Design review of the part built by this model. Coordinates are the model's own, in mm. Face numbers are marked on the shaded views. A direction names the side the tool comes from. Round coordinates to 2 decimals unless told otherwise and drop trailing zeros. Order: outer loops, then holes, each group sorted by start corner. A loop starts at its lowest first (then second) coordinate and runs counter-clockwise, first axis right, second up. Notation, with made-up numbers: M 25.25,46.5 L 40.25,46.5 A8 cw 40.25,55.5 Z; hole C 50,86 d2. An arc over 180 degrees is marked long. Write each question's results on one line, items separated by ' | '. Start each with the question number.
Item 1: The part is to be moulded in two halves that separate along Y. For the marked faces 1, 2 and 3, say which applies: +Y half, -Y half, draft (parallel to the pull), parting line (faces both ways), or undercut.
Item 2: Wall thickness on line 1 (Y direction, x = 15, z = 3.25); line 2 (Z direction, x = 14.5, y = 3); line 3 (Z direction, x = 28.5, y = -6): over which ranges is each line inside the solid? List them lowest first. Write a range as [from, to].
Item 3: Clearance check with flat-ended pins moving along their axes: pin 1 (6 mm diameter, centred on x = -23.5, z = 6.5, fed in from +Y); pin 2 (1 mm diameter, centred on x = 14, y = 1, fed in from +Z); pin 3 (1.2 mm diameter, centred on y = -9.5, z = 3, fed in from -X); pin 4 (2 mm diameter, centred on y = -9, z = 7.5, fed in from -X). State where each tip first meets the part, or that it passes through.
Item 4: Take a section at D-D, the plane z = 3. Write out the cut boundary in (x, y) (3 decimals).
Item 5: Machinability: for the marked faces 4, 5 and 6, which of the approach directions +Z, -Z, +X, -X, +Y, -Y give a long, thin tool a straight path to every point of the face, cutting with its end or side? Answer none if there is none.
Item 6: Take a section at C-C, the plane x = -27. Write out the cut boundary in (y, z).
Item 7: Take a section at A-A, the plane y = 1.25. Write out the cut boundary in (x, z), plus the area to 3 significant figures.
Item 8: Take a section at B-B, the plane z = 6. Write out the cut boundary in (x, y), plus the area to 3 significant figures.
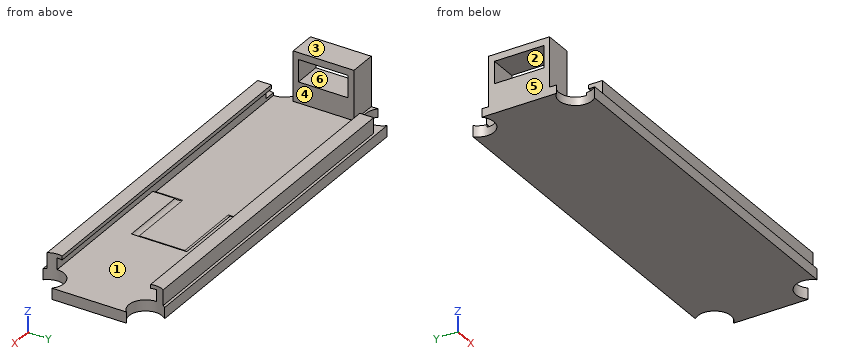
```python
from build123d import *

# Parameters (mm, degrees)
SKIZZE1_W                       = 22
SKIZZE1_H                       = 72.8
AUFSATZ_LINEAR_AUSTRAGEN1_DEPTH = 2
SKIZZE2_R                       = 3
SCHNITT_LINEAR_AUSTRAGEN1_DEPTH = 2
SKIZZE3_W                       = 65.5
SKIZZE3_H                       = 21
AUFSATZ_LINEAR_AUSTRAGEN2_DEPTH = 2.8
SCHNITT_LINEAR_AUSTRAGEN2_DEPTH = 67.590464783
SKIZZE5_R                       = 3
SCHNITT_LINEAR_AUSTRAGEN4_DEPTH = 39.128729326
SKIZZE6_W                       = 18
SKIZZE6_H                       = 1
SCHNITT_LINEAR_AUSTRAGEN5_DEPTH = 40
SKIZZE8_W                       = 15
SKIZZE8_H                       = 10
SCHNITT_LINEAR_AUSTRAGEN6_DEPTH = 0.5
VERRUNDUNG3_R                   = 1
SKIZZE9_W                       = 5
SKIZZE9_H                       = 11
AUFSATZ_LINEAR_AUSTRAGEN3_DEPTH = 9
SKIZZE10_W                      = 9
SKIZZE10_H                      = 4
SCHNITT_LINEAR_AUSTRAGEN7_DEPTH = 75.371298227


with BuildPart() as part:
    # Skizze1 → Aufsatz-Linear austragen1 (new body)
    with BuildSketch(Plane(origin=(0, 0, 0), x_dir=(0, 1, 0), z_dir=(0, 0, 1))):
        Rectangle(SKIZZE1_W, SKIZZE1_H)
    extrude(amount=AUFSATZ_LINEAR_AUSTRAGEN1_DEPTH)

    # Skizze2 → Schnitt-Linear austragen1 (cut)
    with BuildSketch(Plane.XY.offset(2)):
        with Locations((-34.28, 8.88)):
            Circle(SKIZZE2_R)
        with Locations((-34.28, -8.88)):
            Circle(SKIZZE2_R)
        with Locations((34.28, -8.88)):
            Circle(SKIZZE2_R)
        with Locations((34.28, 8.88)):
            Circle(SKIZZE2_R)
    extrude(amount=-SCHNITT_LINEAR_AUSTRAGEN1_DEPTH, mode=Mode.SUBTRACT)

    # Skizze3 → Aufsatz-Linear austragen2 (add)
    with BuildSketch(Plane.XY.offset(2)):
        with Locations((3.65, 0)):
            Rectangle(SKIZZE3_W, SKIZZE3_H)
    extrude(amount=AUFSATZ_LINEAR_AUSTRAGEN2_DEPTH)

    # Skizze4 → Schnitt-Linear austragen2 (cut, through all)
    with BuildSketch(Plane(origin=(-29.1, 0, 0), x_dir=(0, -1, 0), z_dir=(-1, 0, 0))):
        Polygon((-8, 4.8), (8, 4.8), (8, 4.1), (9, 4.1), (9, 2), (-9, 2), (-9, 4.1), (-8, 4.1), align=None)
    extrude(amount=-SCHNITT_LINEAR_AUSTRAGEN2_DEPTH, mode=Mode.SUBTRACT)

    # Skizze5 → Schnitt-Linear austragen4 (cut, through all)
    with BuildSketch(Plane(origin=(0, 0, 2), x_dir=(1, 0, 0), z_dir=(0, 0, -1))):
        with Locations((34.28, -8.88)):
            Circle(SKIZZE5_R)
        with Locations((34.28, 8.88)):
            Circle(SKIZZE5_R)
    extrude(amount=-SCHNITT_LINEAR_AUSTRAGEN4_DEPTH, mode=Mode.SUBTRACT)

    # Skizze6 → Schnitt-Linear austragen5 (cut)
    with BuildSketch(Plane(origin=(-36.4, 0, 0), x_dir=(0, -1, 0), z_dir=(-1, 0, 0))):
        with Locations((0, 2)):
            Rectangle(SKIZZE6_W, SKIZZE6_H)
    extrude(amount=-SCHNITT_LINEAR_AUSTRAGEN5_DEPTH, mode=Mode.SUBTRACT)

    # Skizze8 → Schnitt-Linear austragen6 (cut)
    with BuildSketch(Plane.XY.offset(2)):
        with Locations((8.655984658, -0.007335612)):
            Rectangle(SKIZZE8_W, SKIZZE8_H)
    extrude(amount=-SCHNITT_LINEAR_AUSTRAGEN6_DEPTH, mode=Mode.SUBTRACT)

    # Verrundung3
    # the kernel refuses this fillet: 1 mm, written as the material it adds along each edge
    with BuildSketch(Plane(origin=(3.6, -9, 1.5), x_dir=(0, 0, 1), z_dir=(0, 1, 0))) as verrundung3_piece_1:
        with BuildLine():
            CenterArc((1, -0.866025404), VERRUNDUNG3_R, 120, 60)
            Line((0, -0.866025404), (-0.02, -0.866025404))
            Line((-0.02, -0.866025404), (-0.02, 0))
            Line((-0.02, 0), (0, 0.02))
            ThreePointArc((0, 0.02), (0.25, 0.02), (0.49, 0.017320508))
            Line((0.49, 0.017320508), (0.5, 0))
        make_face()
    extrude(amount=3.992664388)
    with BuildSketch(Plane(origin=(3.6, -5.007335612, 1.5), x_dir=(0, 0, 1), z_dir=(1, 0, 0)), Plane(origin=(16.155984658, 4.992664388, 1.5), x_dir=(0, 0, 1), z_dir=(-1, 0, 0))) as verrundung3_piece_2:
        with BuildLine():
            CenterArc((1, -0.866025404), VERRUNDUNG3_R, 120, 60)
            Line((0, -0.866025404), (-0.02, -0.866025404))
            Line((-0.02, -0.866025404), (-0.02, 0))
            Line((-0.02, 0), (0, 0.02))
            ThreePointArc((0, 0.02), (0.25, 0.02), (0.49, 0.017320508))
            Line((0.49, 0.017320508), (0.5, 0))
        make_face()
    extrude(amount=12.555984658)
    with BuildSketch(Plane(origin=(3.6, 4.992664388, 1.5), x_dir=(0, 0, 1), z_dir=(0, 1, 0))) as verrundung3_piece_3:
        with BuildLine():
            CenterArc((1, -0.866025404), VERRUNDUNG3_R, 120, 60)
            Line((0, -0.866025404), (-0.02, -0.866025404))
            Line((-0.02, -0.866025404), (-0.02, 0))
            Line((-0.02, 0), (0, 0.02))
            ThreePointArc((0, 0.02), (0.25, 0.02), (0.49, 0.017320508))
            Line((0.49, 0.017320508), (0.5, 0))
        make_face()
    extrude(amount=4.007335612)
    with BuildSketch(Plane(origin=(16.155984658, -5.007335612, 1.5), x_dir=(0, 0, 1), z_dir=(0, 1, 0))) as verrundung3_piece_4:
        with BuildLine():
            CenterArc((1, -0.866025404), VERRUNDUNG3_R, 120, 60)
            Line((0, -0.866025404), (-0.02, -0.866025404))
            Line((-0.02, -0.866025404), (-0.02, 0))
            Line((-0.02, 0), (0, 0.02))
            ThreePointArc((0, 0.02), (0.25, 0.02), (0.49, 0.017320508))
            Line((0.49, 0.017320508), (0.5, 0))
        make_face()
    extrude(amount=10)
    with BuildSketch(Plane(origin=(3.6, -9, 1.5), x_dir=(0, 0, 1), z_dir=(0, 1, 0))) as verrundung3_piece_5a_section:
        with BuildLine():
            CenterArc((1, -0.866025404), VERRUNDUNG3_R, 120, 60)
            Line((0, -0.866025404), (-0.02, -0.866025404))
            Line((-0.02, -0.866025404), (-0.02, 0))
            Line((-0.02, 0), (0, 0.02))
            ThreePointArc((0, 0.02), (0.25, 0.02), (0.49, 0.017320508))
            Line((0.49, 0.017320508), (0.5, 0))
        make_face()
    verrundung3_piece_5a = extrude(amount=6.157727897, mode=Mode.PRIVATE)
    verrundung3_piece_5a = split(verrundung3_piece_5a, bisect_by=Plane(origin=(3.383689554, -5.007335612, 1.629516711), z_dir=(0, 1, 0)), keep=Keep.TOP, mode=Mode.PRIVATE)
    with BuildSketch(Plane(origin=(1.434936491, -5.007335612, 1.5), x_dir=(0, 0, 1), z_dir=(1, 0, 0))) as verrundung3_piece_5b_section:
        with BuildLine():
            CenterArc((1, -0.866025404), VERRUNDUNG3_R, 120, 60)
            Line((0, -0.866025404), (-0.02, -0.866025404))
            Line((-0.02, -0.866025404), (-0.02, 0))
            Line((-0.02, 0), (0, 0.02))
            ThreePointArc((0, 0.02), (0.25, 0.02), (0.49, 0.017320508))
            Line((0.49, 0.017320508), (0.5, 0))
        make_face()
    verrundung3_piece_5b = extrude(amount=14.721048168, mode=Mode.PRIVATE)
    verrundung3_piece_5b = split(verrundung3_piece_5b, bisect_by=Plane(origin=(3.6, -4.791025166, 1.629516711), z_dir=(-1, 0, 0)), keep=Keep.TOP, mode=Mode.PRIVATE)
    verrundung3_piece_5 = verrundung3_piece_5a & verrundung3_piece_5b
    add(verrundung3_piece_5)
    with BuildSketch(Plane(origin=(3.6, -5.007335612, 1.5), x_dir=(0, 0, 1), z_dir=(1, 0, 0))) as verrundung3_piece_6a_section:
        with BuildLine():
            CenterArc((1, -0.866025404), VERRUNDUNG3_R, 120, 60)
            Line((0, -0.866025404), (-0.02, -0.866025404))
            Line((-0.02, -0.866025404), (-0.02, 0))
            Line((-0.02, 0), (0, 0.02))
            ThreePointArc((0, 0.02), (0.25, 0.02), (0.49, 0.017320508))
            Line((0.49, 0.017320508), (0.5, 0))
        make_face()
    verrundung3_piece_6a = extrude(amount=14.721048168, mode=Mode.PRIVATE)
    verrundung3_piece_6a = split(verrundung3_piece_6a, bisect_by=Plane(origin=(16.155984658, -4.791025166, 1.629516711), z_dir=(1, 0, 0)), keep=Keep.TOP, mode=Mode.PRIVATE)
    with BuildSketch(Plane(origin=(16.155984658, -7.172399122, 1.5), x_dir=(0, 0, 1), z_dir=(0, 1, 0))) as verrundung3_piece_6b_section:
        with BuildLine():
            CenterArc((1, -0.866025404), VERRUNDUNG3_R, 120, 60)
            Line((0, -0.866025404), (-0.02, -0.866025404))
            Line((-0.02, -0.866025404), (-0.02, 0))
            Line((-0.02, 0), (0, 0.02))
            ThreePointArc((0, 0.02), (0.25, 0.02), (0.49, 0.017320508))
            Line((0.49, 0.017320508), (0.5, 0))
        make_face()
    verrundung3_piece_6b = extrude(amount=12.165063509, mode=Mode.PRIVATE)
    verrundung3_piece_6b = split(verrundung3_piece_6b, bisect_by=Plane(origin=(15.939674213, -5.007335612, 1.629516711), z_dir=(0, -1, 0)), keep=Keep.TOP, mode=Mode.PRIVATE)
    verrundung3_piece_6 = verrundung3_piece_6a & verrundung3_piece_6b
    add(verrundung3_piece_6)
    with BuildSketch(Plane(origin=(16.155984658, 4.992664388, 1.5), x_dir=(0, 0, 1), z_dir=(-1, 0, 0))) as verrundung3_piece_7a_section:
        with BuildLine():
            CenterArc((1, -0.866025404), VERRUNDUNG3_R, 120, 60)
            Line((0, -0.866025404), (-0.02, -0.866025404))
            Line((-0.02, -0.866025404), (-0.02, 0))
            Line((-0.02, 0), (0, 0.02))
            ThreePointArc((0, 0.02), (0.25, 0.02), (0.49, 0.017320508))
            Line((0.49, 0.017320508), (0.5, 0))
        make_face()
    verrundung3_piece_7a = extrude(amount=14.721048168, mode=Mode.PRIVATE)
    verrundung3_piece_7a = split(verrundung3_piece_7a, bisect_by=Plane(origin=(3.6, 4.776353942, 1.629516711), z_dir=(-1, 0, 0)), keep=Keep.TOP, mode=Mode.PRIVATE)
    with BuildSketch(Plane(origin=(3.6, 2.827600878, 1.5), x_dir=(0, 0, 1), z_dir=(0, 1, 0))) as verrundung3_piece_7b_section:
        with BuildLine():
            CenterArc((1, -0.866025404), VERRUNDUNG3_R, 120, 60)
            Line((0, -0.866025404), (-0.02, -0.866025404))
            Line((-0.02, -0.866025404), (-0.02, 0))
            Line((-0.02, 0), (0, 0.02))
            ThreePointArc((0, 0.02), (0.25, 0.02), (0.49, 0.017320508))
            Line((0.49, 0.017320508), (0.5, 0))
        make_face()
    verrundung3_piece_7b = extrude(amount=6.172399122, mode=Mode.PRIVATE)
    verrundung3_piece_7b = split(verrundung3_piece_7b, bisect_by=Plane(origin=(3.383689554, 4.992664388, 1.629516711), z_dir=(0, -1, 0)), keep=Keep.TOP, mode=Mode.PRIVATE)
    verrundung3_piece_7 = verrundung3_piece_7a & verrundung3_piece_7b
    add(verrundung3_piece_7)
    with BuildSketch(Plane(origin=(16.155984658, -5.007335612, 1.5), x_dir=(0, 0, 1), z_dir=(0, 1, 0))) as verrundung3_piece_8a_section:
        with BuildLine():
            CenterArc((1, -0.866025404), VERRUNDUNG3_R, 120, 60)
            Line((0, -0.866025404), (-0.02, -0.866025404))
            Line((-0.02, -0.866025404), (-0.02, 0))
            Line((-0.02, 0), (0, 0.02))
            ThreePointArc((0, 0.02), (0.25, 0.02), (0.49, 0.017320508))
            Line((0.49, 0.017320508), (0.5, 0))
        make_face()
    verrundung3_piece_8a = extrude(amount=12.165063509, mode=Mode.PRIVATE)
    verrundung3_piece_8a = split(verrundung3_piece_8a, bisect_by=Plane(origin=(15.939674213, 4.992664388, 1.629516711), z_dir=(0, 1, 0)), keep=Keep.TOP, mode=Mode.PRIVATE)
    with BuildSketch(Plane(origin=(18.321048168, 4.992664388, 1.5), x_dir=(0, 0, 1), z_dir=(-1, 0, 0))) as verrundung3_piece_8b_section:
        with BuildLine():
            CenterArc((1, -0.866025404), VERRUNDUNG3_R, 120, 60)
            Line((0, -0.866025404), (-0.02, -0.866025404))
            Line((-0.02, -0.866025404), (-0.02, 0))
            Line((-0.02, 0), (0, 0.02))
            ThreePointArc((0, 0.02), (0.25, 0.02), (0.49, 0.017320508))
            Line((0.49, 0.017320508), (0.5, 0))
        make_face()
    verrundung3_piece_8b = extrude(amount=14.721048168, mode=Mode.PRIVATE)
    verrundung3_piece_8b = split(verrundung3_piece_8b, bisect_by=Plane(origin=(16.155984658, 4.776353942, 1.629516711), z_dir=(1, 0, 0)), keep=Keep.TOP, mode=Mode.PRIVATE)
    verrundung3_piece_8 = verrundung3_piece_8a & verrundung3_piece_8b
    add(verrundung3_piece_8)

    # Skizze9 → Aufsatz-Linear austragen3 (add)
    with BuildSketch(Plane.XY.offset(1.5)):
        with Locations((-33.9, 0)):
            Rectangle(SKIZZE9_W, SKIZZE9_H)
    extrude(amount=AUFSATZ_LINEAR_AUSTRAGEN3_DEPTH)

    # Skizze10 → Schnitt-Linear austragen7 (cut, through all)
    with BuildSketch(Plane(origin=(-36.4, 0, 0), x_dir=(0, -1, 0), z_dir=(-1, 0, 0))):
        with Locations((0.038201858, 7.263431172)):
            Rectangle(SKIZZE10_W, SKIZZE10_H)
    extrude(amount=-SCHNITT_LINEAR_AUSTRAGEN7_DEPTH, mode=Mode.SUBTRACT)


solid = part.part
```
Results list:
1) face 1: undercut | face 2: undercut | face 3: draft
2) line 1: [-10.5, -9], [9, 10.5] | line 2: [0, 1.5] | line 3: [0, 2]
3) pin 1: y = 10.5 | pin 2: z = 1.5 | pin 3: x = -29.1 | pin 4: through
4) outline: M -36.4,-5.5 L -31.4,-5.5 L -31.4,5.5 L -36.4,5.5 Z; M -29.1,-10.5 L 31.755,-10.5 A3 cw 31.282,-9 L -29.1,-9 Z; M -29.1,9 L 31.282,9 A3 cw 31.755,10.5 L -29.1,10.5 Z
5) face 4: +Z | face 5: +Z, -Z, -X, +Y, -Y | face 6: +X, -X
6) outline: M -11,0 L 11,0 L 11,2 L 10.5,2 L 10.5,4.8 L 8,4.8 L 8,4.1 L 9,4.1 L 9,1.5 L -9,1.5 L -9,4.1 L -8,4.1 L -8,4.8 L -10.5,4.8 L -10.5,2 L -11,2 Z
7) outline: M -36.4,0 L 36.4,0 L 36.4,2 L 16.16,2 A1 cw 15.29,1.5 L -31.4,1.5 L -31.4,5.26 L -36.4,5.26 Z; M -36.4,9.26 L -31.4,9.26 L -31.4,10.5 L -36.4,10.5 Z | area: 144 mm²
8) outline: M -36.4,-5.5 L -31.4,-5.5 L -31.4,-4.54 L -36.4,-4.54 Z; M -36.4,4.46 L -31.4,4.46 L -31.4,5.5 L -36.4,5.5 Z | area: 10.0 mm²
